For this review, use the dimensioned drawing (mm, ordinates from the lowest corner) and the shaded views. A direction names the side the tool comes from. Give positions to 0.01 mm unless a question says otherwise; leave off trailing zeros. Loops run counter-clockwise (first coordinate to the right, second up) from the corner with the lowest first, then second, coordinate; pieces in that order, holes last. Notation, with made-up numbers: (-22, 12.5) -> (29, 12.5) arc R24 ccw to (29, 43.5) -> close; hole circle Ø3 at (-15.75, 81). An arc over 180 degrees is marked (long way). Use a Markdown table: item, result. Add a question column.
1. For the marked faces 1, 2, 3, 4 and 5, list the 3-axis set-ups (+Z, -Z, +X, -X, +Y, -Y) from which the entire face can be reached by the end or side of a thin tool; tool diameter is ignored.
2. Add section D-D (x = 1.5). State the section outline as (y, z) points (1 decimal).
3. To check wall thickness, follow line 1 (Y direction, x = 0.75, z = 1.3) (1 decimal); line 2 (Y direction, x = 4.75, z = 2.8) (1 decimal); line 3 (Y direction, x = 5.75, z = 0.3) (1 decimal). State the ranges of each line that lie inside material, in increasing order.
4. Draft analysis for pull direction X (two halves, no side actions). For the marked faces 6, 7 and 8, state which applies: pulls with the +X half, pulls with the -X half, needs draft (parallel to the pull), parting line crosses it, or undercut.
5. For pin 1 Ø1.5 at (x, y) = (1, 8.5) entering from +Z; pin 2 Ø2.5 at (x, z) = (4.5, 2.5) entering from -Y; pin 3 Ø0.8 at (x, z) = (6, 2) entering from +Y; pin 4 Ø0.8 at (y, z) = (8, 3.5) entering from -X, all flat-tipped, find the tip position at first contact; note any pin that passes through.
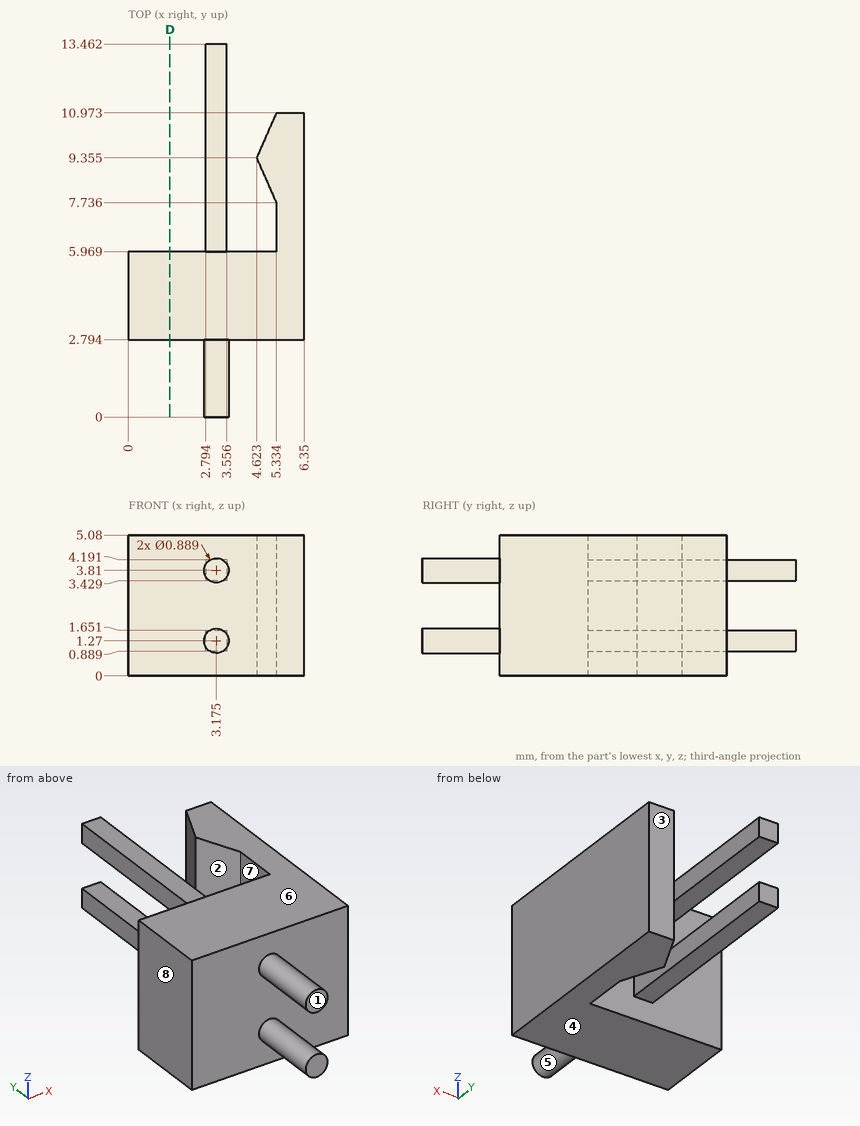
Taken from the geometry:
| question | item | result |
|---|---|---|
| 1 | face 1 | +Z, -Z, +X, -X, -Y |
| 1 | face 2 | +Z, -Z |
| 1 | face 3 | +Z, -Z, +X, +Y |
| 1 | face 4 | -Z, +X, -X, +Y, -Y |
| 1 | face 5 | -Y |
| 2 | outline | (2.8, 0) -> (6, 0) -> (6, 5.1) -> (2.8, 5.1) -> close |
| 3 | line 1 | y = 2.8 to 6 |
| 3 | line 2 | y = 2.8 to 6, 9.1 to 9.6 |
| 3 | line 3 | y = 2.8 to 11 |
| 4 | face 6 | needs draft |
| 4 | face 7 | undercut |
| 4 | face 8 | pulls with the -X half |
| 5 | pin 1 | passes through |
| 5 | pin 2 | stops at y = 2.79 |
| 5 | pin 3 | stops at y = 10.97 |
| 5 | pin 4 | stops at x = 2.79 |
